Part model, mm, in its own coordinate system. A direction names the side the tool comes from. Coordinates: 2 decimals unless noted, no trailing zeros. Order: outer loops, then holes, each group sorted by start corner. A loop starts at its lowest first (then second) coordinate and runs counter-clockwise, first axis right, second up. Notation, with made-up numbers: M 73,37.5 L 93,37.5 A27 ccw 93,68.5 Z; hole C -19.5,-3.5 d4. An arc over 180 degrees is marked long. Write item = value, one per line. Start each with the question number.
from build123d import *

# Parameters (mm, degrees)
SKETCH1_W           = 140
SKETCH1_H           = 80
BOSS_EXTRUDE1_DEPTH = 20
BOSS_EXTRUDE2_DEPTH = 80
SKETCH3_W           = 2.5
SKETCH3_H           = 40
SKETCH4_R           = 9
CUT_EXTRUDE1_DEPTH  = 125.510684884


with BuildPart() as part:
    # Sketch1 → Boss-Extrude1 (new body)
    with BuildSketch(Plane(origin=(0, 0, 0), x_dir=(1, 0, 0), z_dir=(0, 1, 0))):
        Rectangle(SKETCH1_W, SKETCH1_H)
    extrude(amount=BOSS_EXTRUDE1_DEPTH)

    # Sketch2 → Boss-Extrude2 (add, through all)
    with BuildSketch(Plane.XY.offset(40)):
        with BuildLine():
            Line((30, 94.883669039), (50, 94.883669039))
            Line((50, 94.883669039), (50, 20))
            Line((50, 20), (-50, 20))
            Line((-50, 20), (-50, 94.883669039))
            Line((-50, 94.883669039), (-30, 94.883669039))
            ThreePointArc((-30, 94.883669039), (0, 64.883669039), (30, 94.883669039))
        make_face()
    extrude(amount=-BOSS_EXTRUDE2_DEPTH)

    # Sketch3 → Cut-Revolve1 (revolve, cut)
    with BuildSketch(Plane(origin=(0, 94.883669039, 0), x_dir=(1, 0, 0), z_dir=(0, 1, 0))):
        with Locations((-31.25, 0)):
            Rectangle(SKETCH3_W, SKETCH3_H)
    revolve(axis=Axis((0, 94.883669039, 29.575987761), (0, 0, -1)), mode=Mode.SUBTRACT)

    # Sketch4 → Cut-Extrude1 (cut, through all)
    with BuildSketch(Plane(origin=(0, 94.883669039, 0), x_dir=(1, 0, 0), z_dir=(0, 1, 0))):
        with Locations(Location((50, 0, 0), (0, 0, 270))):
            Circle(SKETCH4_R)
    cut_extrude1 = extrude(amount=-CUT_EXTRUDE1_DEPTH, mode=Mode.SUBTRACT)

    # Mirror1: Cut-Extrude1 across plane
    add(cut_extrude1.mirror(Plane(origin=(0, 0, 0), x_dir=(0, 0, 1), z_dir=(1, 0, 0))), mode=Mode.SUBTRACT)


solid = part.part
Item 1: Cut at C-C, the plane z = -7. Write the cut outline in (x, y).
Item 2: Cut at B-B, the plane y = 15. Write the cut outline in (x, z), and give its area (3 significant figures).
Item 3: 3-axis set-ups, long thin cutter, end or side, ignore diameter. For faces 1 (the flat face through (50, 58, 25)), 2 (the flat face through (40, 94.884, 1)), 3 (the flat face through (0, 64, -20)), 4 (the flat face through (-50, 57, -24)): which of +Z, -Z, +X, -X, +Y, -Y reach the whole face in a straight line?
Item 4: Flat gauge pins, fed straight in: pin 1 (1.5 mm diameter, centred on x = 13.5, y = 70, fed in from -Z); pin 2 (25 mm diameter, centred on y = 59, z = -24.5, fed in from -X); pin 3 (15.5 mm diameter, centred on y = 46.5, z = -20, fed in from +X); pin 4 (8 mm diameter, centred on x = -7.5, z = 31, fed in from +Y). Where does each tip first touch, or does it go through?
Item 5: Cut at D-D, the plane z = -24. Write the cut outline in (x, y).
Item 6: Wall check: line 1 along X through (y, z) = (6, 7); line 2 along Z through (x, y) = (47, 38); line 3 along X through (y, z) = (30, 0). Give the ranges that are in metal, low to high. Write a range as [from, to].
Item 7: Cut at A-A, the plane x = 0. Write the cut outline in (y, z), and give its area (3 significant figures).
Item 8: Pull direction Z, two halves, no side cores. Call faces 5 (the flat face through (-1, 36, -40)), 6 (the cylindrical face through (0.71, 62.39, -0.28)), 7 (the flat face through (-50, 57, 25)): pulls with the +Z half, pulls with the -Z half, needs draft (parallel to the pull), parting line crosses it, or undercut.
Filled sheet:
q1.outline = M -70,0 L -55.66,0 L -55.66,20 L -70,20 Z; M -44.34,0 L 44.34,0 L 44.34,94.88 L 32.5,94.88 A32.5 cw -32.5,94.88 L -44.34,94.88 Z; M 55.66,0 L 70,0 L 70,20 L 55.66,20 Z
q2.outline = M -70,-40 L 70,-40 L 70,40 L -70,40 Z; hole C -50,0 d18; hole C 50,0 d18
q2.area = 10,700 mm2
q3.face_1 = +Z, -Z, +X, +Y
q3.face_2 = +Z, -Z, +X, -X, +Y
q3.face_3 = +Y
q3.face_4 = +Z, -Z, -X, +Y
q4.pin_1 = through
q4.pin_2 = -50
q4.pin_3 = 50
q4.pin_4 = 67.18
q5.outline = M -70,0 L 70,0 L 70,20 L 50,20 L 50,94.88 L 30,94.88 A30 cw -30,94.88 L -50,94.88 L -50,20 L -70,20 Z
q6.line_1 = [-70, -55.66], [-44.34, 44.34], [55.66, 70]
q6.line_2 = [-40, -8.49], [8.49, 40]
q6.line_3 = [-41, 41]
q7.outline = M 0,-40 L 64.88,-40 L 64.88,-20 L 62.38,-20 L 62.38,20 L 64.88,20 L 64.88,40 L 0,40 Z
q7.area = 5,090 mm2
q8.face_5 = pulls with the -Z half
q8.face_6 = undercut
q8.face_7 = needs draft
